Work out the finished part from the listing and answer in its coordinate system (mm). Face numbers are marked on the shaded views. Round coordinates to 2 decimals unless told otherwise and drop trailing zeros. Loops run counter-clockwise (first coordinate to the right, second up) from the corner with the lowest first, then second, coordinate; pieces in that order, holes last. Notation, with made-up numbers: (71, 68) - (82, 68) arc R20 cw to (82, 97) - close; hole circle Ø3 at (80.5, -29.75). An arc over 180 degrees is marked (long way). Return JSON: item names as keys, results as strings.
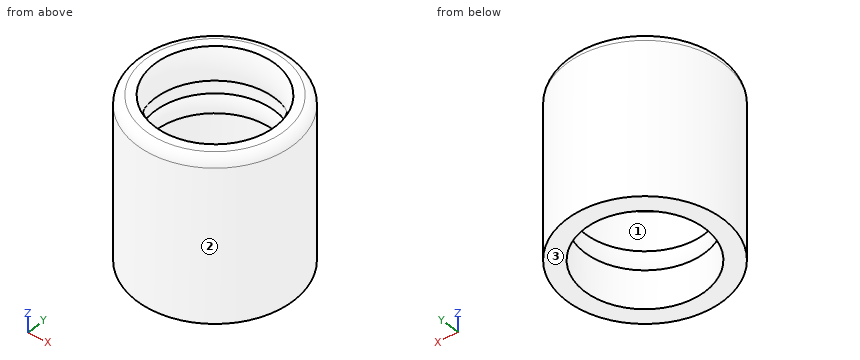
from build123d import *

# Parameters (mm, degrees)
F2_R = 3


with BuildPart() as f1:
    # F0 (on Front) → F1 (revolve)
    with BuildSketch(Plane.XZ):
        with BuildLine():
            ThreePointArc((-20, 52.662842), (-18.333853, 58.331421), (-20, 64))
            Line((-20, 64), (-26, 64))
            Line((-26, 64), (-26, 10))
            Line((-26, 10), (-20, 10))
            Line((-20, 10), (-20, 22.722758))
            ThreePointArc((-20, 22.722758), (-18.82131, 25.840918), (-20, 28.959077))
            Line((-20, 28.959077), (-20, 41.979928))
            ThreePointArc((-20, 41.979928), (-18.710805, 45.238344), (-20, 48.49676))
            Line((-20, 48.49676), (-20, 52.662842))
        make_face()
    revolve(axis=Axis((0, 0, 15.521475), (0, 0, -1)))

    # F2
    f2_edges = [f1.edges().sort_by_distance(p)[0] for p in [
        (26, 0, 64),
    ]]
    fillet(f2_edges, radius=F2_R)


solid = f1.part
1) Section C-C (z = 32.5) is taken. Give the vertices of the cut face in (x, y), and give its area (3 significant figures).
Verdict:
{"outline": "circle Ø52 at (0, 0); hole circle Ø40 at (0, 0)", "area": "867 mm2"}
2) Find the intervals of material crossed by L1, parallel to Y at x = 0, z = 14; L2, parallel to Y at x = -8, z = 58; L3, parallel to X at y = 3.5, z = 46, in increasing order.
Verdict:
{"L1": "y = -26 to -20, 20 to 26", "L2": "y = -24.74 to -16.5, 16.5 to 24.74", "L3": "x = -25.76 to -18.44, 18.44 to 25.76"}
3) Determine the mould class of the marked faces 1, 2 and 3 for opening direction Y: pulls with the +Y half, pulls with the -Y half, needs draft (parallel to the pull), parting line crosses it, or undercut.
Verdict:
{"face 1": "undercut", "face 2": "parting line crosses it", "face 3": "needs draft"}
4) Flat-ended cylindrical pins translate along their axes: pin 1 (1 mm diameter, centred on x = 0.5, z = 17, fed in from -Y); pin 2 (1.5 mm diameter, centred on x = -0.5, y = 18.5, fed in from +Z); pin 3 (2 mm diameter, centred on y = 3, z = 32, fed in from +X). Find the tip coordinate at first contact, or state that the pin passes through.
Verdict:
{"pin 1": "stops at y = -26", "pin 2": "stops at z = 62.63", "pin 3": "stops at x = 25.92"}
5) Section D-D (z = 25) is taken. Give the vertices of the cut face in (x, y), and give its area (3 significant figures).
Verdict:
{"outline": "circle Ø52 at (0, 0); hole circle Ø37.79 at (0, 0)", "area": "1,000 mm2"}
6) Section A-A (y = 0) is taken. Give the vertices of the cut face in (x, z), and give its area (3 significant figures).
Verdict:
{"outline": "(-26, 10) - (-20, 10) - (-20, 22.72) arc R4.71 ccw to (-20, 28.96) - (-20, 41.98) arc R4.76 ccw to (-20, 48.5) - (-20, 52.66) arc R10.48 ccw to (-20, 64) - (-23, 64) arc R3 ccw to (-26, 61) - close; (20, 10) - (26, 10) - (26, 61) arc R3 ccw to (23, 64) - (20, 64) arc R10.48 ccw to (20, 52.66) - (20, 48.5) arc R4.76 ccw to (20, 41.98) - (20, 28.96) arc R4.71 ccw to (20, 22.72) - close", "area": "691 mm2"}
